Verification items for this drawing (mm, ordinates from the low corner). A direction names the side the tool comes from. Coordinates: 2 decimals unless noted, no trailing zeros. Write each loop counter-clockwise with the first axis right and the second up, starting at its lowest first coordinate (ties: lowest second). Pieces come first, ordered by that corner, then holes. Notation, with made-up numbers: (54, -36.5) -> (60, -36.5) arc R8 ccw to (60, -26.5) -> close; hole circle Ø8 at (63.5, 14). An arc over 180 degrees is marked (long way). One line per question, with ' | ' between items.
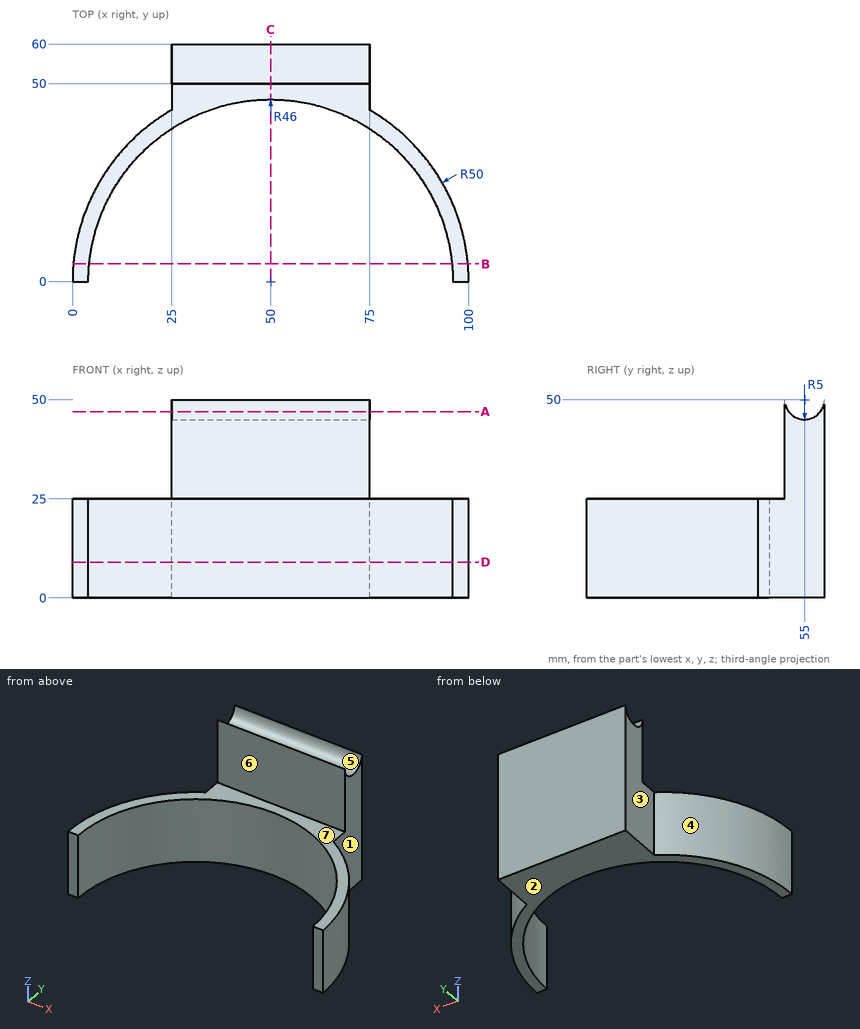
(1) Draft check along Y on the marked faces 4, 5, 6 and 7. Enter one of: pulls with the +Y half, pulls with the -Y half, needs draft (parallel to the pull), parting line crosses it, or undercut.
Answers below:
face 4: pulls with the +Y half | face 5: undercut | face 6: pulls with the -Y half | face 7: needs draft
(2) Depth check by flat-ended pin: P1, Ø5, axis at y = 48, z = 23.5, coming from the +X side; P2, Ø6, axis at x = 42, z = 11, coming from the -Y side; P3, Ø7.5, axis at x = 40, z = 33, coming from the -Y side. Enter the tip coordinate at first touch or a pass-through.
Answers below:
P1: stops at x = 75 | P2: stops at y = 44.67 | P3: stops at y = 50
(3) Cross-section at C-C (x = 50). Record the cut outline in (y, z), plus the area to 3 significant figures.
Answers below:
outline: (46, 0) -> (60, 0) -> (60, 50) arc R5 cw to (50, 50) -> (50, 25) -> (46, 25) -> close | area: 561 mm²
(4) Tool access check on the marked faces 1, 2 and 3. Record the directions out of +Z, -Z, +X, -X, +Y, -Y that give a thin tool (end or side, any length) a straight path to the whole face; none if there is none.
Answers below:
face 1: +Z, -Z, +X, +Y | face 2: -Z, +X, -X, +Y, -Y | face 3: +Z, -Z, -X, +Y
(5) Cross-section at D-D (z = 9). Record the cut outline in (x, y), plus the area to 3 significant figures.
Answers below:
outline: (0, 0) -> (4, 0) arc R46 cw to (96, 0) -> (100, 0) arc R50 ccw to (75, 43.3) -> (75, 60) -> (25, 60) -> (25, 43.3) arc R50 ccw to start | area: 1,210 mm²
(6) Cross-section at B-B (y = 4.5). Record the cut outline in (x, z), plus the area to 3 significant figures.
Answers below:
outline: (0.2, 0) -> (4.22, 0) -> (4.22, 25) -> (0.2, 25) -> close; (95.78, 0) -> (99.8, 0) -> (99.8, 25) -> (95.78, 25) -> close | area: 201 mm²
(7) Cross-section at A-A (z = 47). Record the cut outline in (x, y).
Answers below:
outline: (25, 50) -> (75, 50) -> (75, 51) -> (25, 51) -> close; (25, 59) -> (75, 59) -> (75, 60) -> (25, 60) -> close
(8) Material ranges on line 1 (Y direction, x = 64.5, z = 34.5); line 2 (X direction, y = 47, z = 15); line 3 (Z direction, x = 12.5, y = 30.5), recorded low to high.
Answers below:
line 1: y = 50 to 60 | line 2: x = 25 to 75 | line 3: z = 0 to 25
